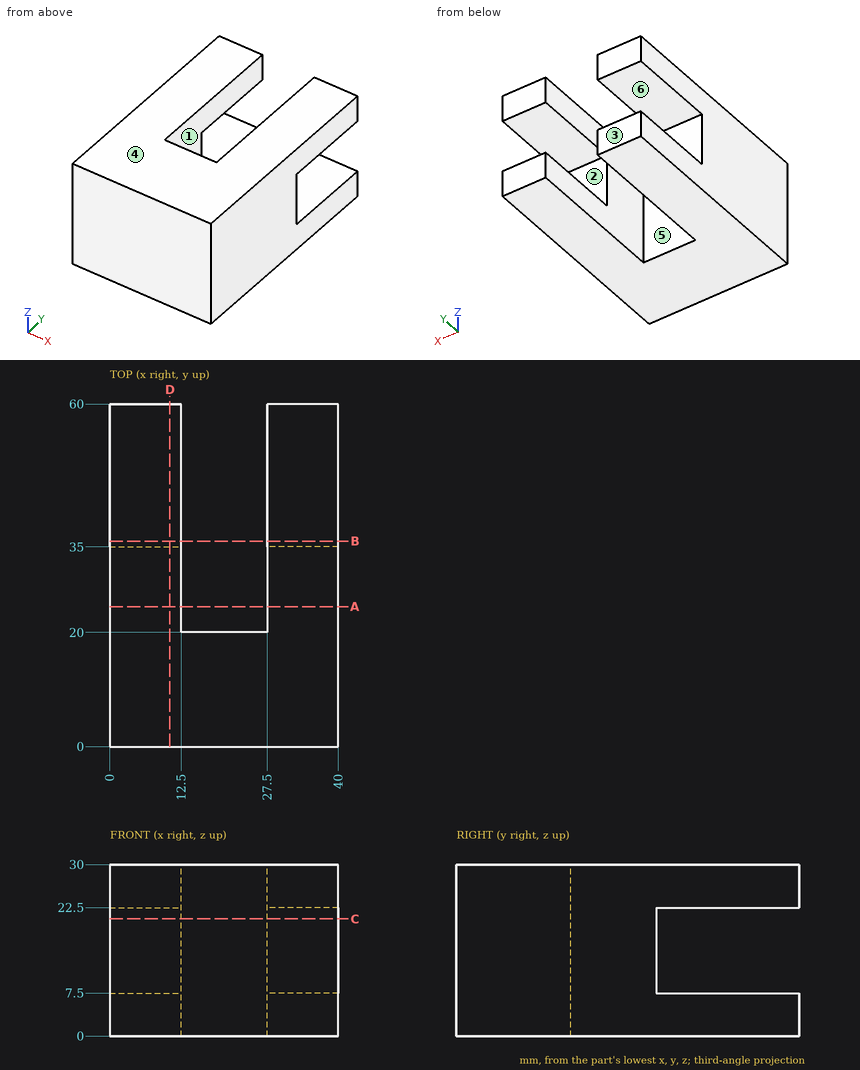
Verification items for this drawing (mm, ordinates from the low corner). A direction names the side the tool comes from. Give positions to 0.01 mm unless a question says otherwise; leave off trailing zeros. Loops run counter-clockwise (first coordinate to the right, second up) from the corner with the lowest first, then second, coordinate; pieces in that order, holes last. Notation, with made-up numbers: M -3,-4 L 4,-4 A25 ccw 4,31 Z; hole C 46,46 d9. An arc over 180 degrees is marked long. Answer as a JSON object with one key per item and string values. Group by question number.
Item 1: Access from +Z, -Z, +X, -X, +Y, -Y to the whole of each face (thin tool, end or side, straight path). Record for the marked faces 1, 2 and 3.
Item 2: Sectioned sample at A-A on y = 24.5. Record the boundary of the cut face in (x, z).
Item 3: Sectioned sample at C-C on z = 20.5. Record the boundary of the cut face in (x, y), plus the area to 4 significant figures.
Item 4: Material ranges on L1, parallel to Z at x = 31.5, y = 56; L2, parallel to X at y = 47, z = 24; L3, parallel to Y at x = 13.5, z = 5.5, recorded low to high.
Item 5: Sectioned sample at B-B on y = 36. Record the boundary of the cut face in (x, z).
Item 6: Mould release check, pull along Z, two halves, no side actions. Record for the marked faces 4, 5 and 6: pulls with the +Z half, pulls with the -Z half, needs draft (parallel to the pull), parting line crosses it, or undercut.
Item 7: Gauge pin test, flat end, axial feed: pin 1 (4 mm diameter, centred on x = 32.5, z = 18.5, fed in from +Y). Record the tip position at first contact, or that the pin passes through.
Item 8: Sectioned sample at D-D on x = 10.5. Record the boundary of the cut face in (y, z), plus the area to 4 significant figures.
Findings below:
{
 "1": {"face 1": "+Z, -Z, +Y", "face 2": "+X, -X, +Y", "face 3": "+Z, -Z, +X, -X, +Y"},
 "2": {"outline": "M 0,0 L 12.5,0 L 12.5,30 L 0,30 Z; M 27.5,0 L 40,0 L 40,30 L 27.5,30 Z"},
 "3": {"outline": "M 0,0 L 40,0 L 40,35 L 27.5,35 L 27.5,20 L 12.5,20 L 12.5,35 L 0,35 Z", "area": "1,175 mm2"},
 "4": {"L1": "0 to 7.5, 22.5 to 30", "L2": "0 to 12.5, 27.5 to 40", "L3": "0 to 20"},
 "5": {"outline": "M 0,0 L 12.5,0 L 12.5,7.5 L 0,7.5 Z; M 0,22.5 L 12.5,22.5 L 12.5,30 L 0,30 Z; M 27.5,0 L 40,0 L 40,7.5 L 27.5,7.5 Z; M 27.5,22.5 L 40,22.5 L 40,30 L 27.5,30 Z"},
 "6": {"face 4": "pulls with the +Z half", "face 5": "needs draft", "face 6": "undercut"},
 "7": {"pin 1": "y = 35"},
 "8": {"outline": "M 0,0 L 60,0 L 60,7.5 L 35,7.5 L 35,22.5 L 60,22.5 L 60,30 L 0,30 Z", "area": "1,425 mm2"}
}
